```python
from build123d import *

# Parameters (mm, degrees)
SKETCH1_R                      = 1.35
BASE_FLANGE1_DEPTH             = 0.8
EDGE_FLANGE1_STRIP_W           = 7.2
EDGE_FLANGE1_STRIP_H           = 0.8
EDGE_FLANGE1_STRIP_CUT_DEPTH   = 50
EDGE_FLANGE1_STRIP_2_W         = 7.2
EDGE_FLANGE1_STRIP_2_H         = 0.8
EDGE_FLANGE1_STRIP_CUT_2_DEPTH = 55.5
EDGE_FLANGE1_DEPTH             = 50
EDGE_FLANGE1_BEND_DEPTH        = 55.5
EDGE_FLANGE4_DEPTH             = 11.5
EDGE_FLANGE4_BEND_DEPTH        = 11.5
EDGE_FLANGE5_DEPTH             = 50
EDGE_FLANGE5_BEND_DEPTH        = 55.5


# Sheet-metal steps are written as plain solids
with BuildPart() as part:
    # Sketch1 → Base-Flange1 (new body)
    with BuildSketch(Plane.XY):
        Polygon((16.25, 0), (16.25, -17), (-14.25, -17), (-14.25, -5.5), (-23.25, -5.5), (-23.25, 50), (-14.25, 50), (-14.25, 65), (16.25, 65), (16.25, 50), (21.25, 50), (21.25, 0), align=None)
        with Locations((9.737756115, -14)):
            Circle(SKETCH1_R, mode=Mode.SUBTRACT)
        with Locations((-4.262243885, -14)):
            Circle(SKETCH1_R, mode=Mode.SUBTRACT)
        with Locations((9.737756115, 62)):
            Circle(SKETCH1_R, mode=Mode.SUBTRACT)
        with Locations((-4.262243885, 62)):
            Circle(SKETCH1_R, mode=Mode.SUBTRACT)
    extrude(amount=BASE_FLANGE1_DEPTH)

    # Edge-Flange1 strip (across the edge) → Edge-Flange1 strip cut (cut)
    with BuildSketch(Plane(origin=(21.25, 50, 0), x_dir=(-1, 0, 0), z_dir=(0, -1, 0))):
        with Locations((-1.6, -0.4)):
            Rectangle(EDGE_FLANGE1_STRIP_W, EDGE_FLANGE1_STRIP_H)
    extrude(amount=EDGE_FLANGE1_STRIP_CUT_DEPTH, mode=Mode.SUBTRACT)

    # Edge-Flange1 strip 2 (across the edge) → Edge-Flange1 strip cut 2 (cut)
    with BuildSketch(Plane(origin=(-23.25, -5.5, 0), x_dir=(1, 0, 0), z_dir=(0, 1, 0))):
        with Locations((-1.6, -0.4)):
            Rectangle(EDGE_FLANGE1_STRIP_2_W, EDGE_FLANGE1_STRIP_2_H)
    extrude(amount=EDGE_FLANGE1_STRIP_CUT_2_DEPTH, mode=Mode.SUBTRACT)

    # Edge-Flange1 section (across the edge) → Edge-Flange1 (add)
    with BuildSketch(Plane(origin=(21.25, 50, 0), x_dir=(-1, 0, 0), z_dir=(0, -1, 0))):
        with BuildLine():
            Line((-0.8, 2), (-0.8, 13.5))
            Line((-0.8, 13.5), (0, 13.5))
            Line((0, 13.5), (0, 2))
            ThreePointArc((0, 2), (0.585786438, 0.585786438), (2, 0))
            Line((2, 0), (2, -0.8))
            ThreePointArc((2, -0.8), (0.020101013, 0.020101013), (-0.8, 2))
        make_face()
    extrude(amount=EDGE_FLANGE1_DEPTH)

    # Edge-Flange1 section 2 (across the edge) → Edge-Flange1 bend (add)
    with BuildSketch(Plane(origin=(-23.25, -5.5, 0), x_dir=(1, 0, 0), z_dir=(0, 1, 0))):
        with BuildLine():
            Line((-0.8, 2), (-0.8, 13.5))
            Line((-0.8, 13.5), (0, 13.5))
            Line((0, 13.5), (0, 2))
            ThreePointArc((0, 2), (0.585786438, 0.585786438), (2, 0))
            Line((2, 0), (2, -0.8))
            ThreePointArc((2, -0.8), (0.020101013, 0.020101013), (-0.8, 2))
        make_face()
    extrude(amount=EDGE_FLANGE1_BEND_DEPTH)

    # Edge-Flange4 section (across the edge) → Edge-Flange4 (add)
    with BuildSketch(Plane(origin=(21.25, 52, -2), x_dir=(0, -1, 0), z_dir=(0, 0, -1))):
        with BuildLine():
            Line((-0.8, 2), (-0.8, 20))
            Line((-0.8, 20), (0, 20))
            Line((0, 20), (0, 2))
            ThreePointArc((0, 2), (0.585786438, 0.585786438), (2, 0))
            Line((2, 0), (2, -0.8))
            ThreePointArc((2, -0.8), (0.020101013, 0.020101013), (-0.8, 2))
        make_face()
    extrude(amount=EDGE_FLANGE4_DEPTH)

    # Edge-Flange4 section 2 (across the edge) → Edge-Flange4 bend (add)
    with BuildSketch(Plane(origin=(-23.25, 52, -13.5), x_dir=(0, -1, 0), z_dir=(0, 0, 1))):
        with BuildLine():
            Line((-0.8, 2), (-0.8, 20))
            Line((-0.8, 20), (0, 20))
            Line((0, 20), (0, 2))
            ThreePointArc((0, 2), (0.585786438, 0.585786438), (2, 0))
            Line((2, 0), (2, -0.8))
            ThreePointArc((2, -0.8), (0.020101013, 0.020101013), (-0.8, 2))
        make_face()
    extrude(amount=EDGE_FLANGE4_BEND_DEPTH)

    # Edge-Flange5 section (across the edge) → Edge-Flange5 (add)
    with BuildSketch(Plane(origin=(21.25, 50, -15.5), x_dir=(0, 0, 1), z_dir=(0, -1, 0))):
        with BuildLine():
            Line((-0.8, 2), (-0.8, 10))
            Line((-0.8, 10), (0, 10))
            Line((0, 10), (0, 2))
            ThreePointArc((0, 2), (0.585786438, 0.585786438), (2, 0))
            Line((2, 0), (2, -0.8))
            ThreePointArc((2, -0.8), (0.020101013, 0.020101013), (-0.8, 2))
        make_face()
    extrude(amount=EDGE_FLANGE5_DEPTH)

    # Edge-Flange5 section 2 (across the edge) → Edge-Flange5 bend (add)
    with BuildSketch(Plane(origin=(-23.25, -5.5, -15.5), x_dir=(0, 0, 1), z_dir=(0, 1, 0))):
        with BuildLine():
            Line((-0.8, 2), (-0.8, 10))
            Line((-0.8, 10), (0, 10))
            Line((0, 10), (0, 2))
            ThreePointArc((0, 2), (0.585786438, 0.585786438), (2, 0))
            Line((2, 0), (2, -0.8))
            ThreePointArc((2, -0.8), (0.020101013, 0.020101013), (-0.8, 2))
        make_face()
    extrude(amount=EDGE_FLANGE5_BEND_DEPTH)


solid = part.part
```
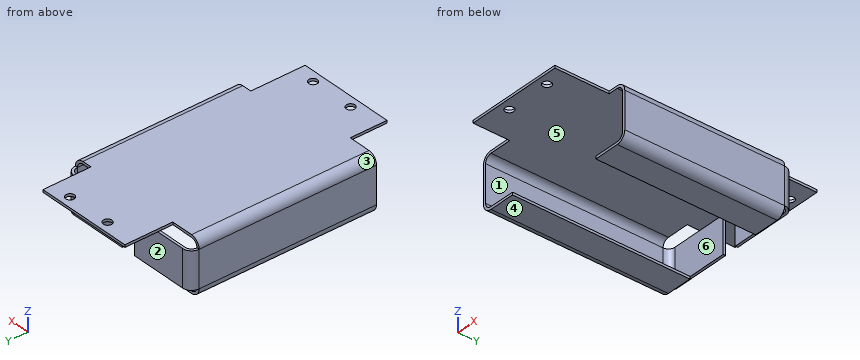
Work out the finished part from the listing and answer in its coordinate system (mm). Face numbers are marked on the shaded views. A direction names the side the tool comes from. Give positions to 0.01 mm unless a question says otherwise; leave off trailing zeros. Loops run counter-clockwise (first coordinate to the right, second up) from the corner with the lowest first, then second, coordinate; pieces in that order, holes last. Notation, with made-up numbers: (61, 30) -> (114, 30) arc R10 cw to (114, 35) -> close; hole circle Ø6 at (-4.5, 84.25). An arc over 180 degrees is marked (long way). Use CSV: the item, a comma, the result in double quotes.
1. A tool of negligible diameter and unlimited length cuts with its end or side. For the marked faces 4, 5 and 6, from which of +Z, -Z, +X, -X, +Y, -Y can it reach the whole face along a straight path? Write none if from no direction.
Found:
face 4,"-Z, +X, -X, +Y, -Y"
face 5,"+Y, -Y"
face 6,"-Z, -Y"
2. The part is cut by section A-A (x = -10.5). Write down the section's boundary in (y, z), then the cut area to 3 significant figures.
Found:
outline,"(-17, 0) -> (65, 0) -> (65, 0.8) -> (-17, 0.8) -> close; (52, -13.5) -> (52.8, -13.5) -> (52.8, -2) -> (52, -2) -> close"
area,"74.8 mm^2"
3. Straight lines are drawn through the part: line 1 (X direction, y = 47.5, z = -4.5); line 2 (Y direction, x = 6.5, z = -6.25); line 3 (Z direction, x = 7, y = 49). For each, find the intervals that lie inside material, in ascending order.
Found:
line 1,"-24.05 to -23.25, 21.25 to 22.05"
line 2,"52 to 52.8"
line 3,"0 to 0.8"
4. The mould has two halves that part along Z. Classify the marked faces 1, 2 and 3: +Z half, -Z half, draft (parallel to the pull), parting line (faces both ways), or undercut.
Found:
face 1,"undercut"
face 2,"draft"
face 3,"+Z half"
5. The part is cut by section B-B (y = 62). Write down the section's boundary in (x, z), then the cut area to 3 significant figures.
Found:
outline,"(-14.25, 0) -> (-5.61, 0) -> (-5.61, 0.8) -> (-14.25, 0.8) -> close; (-2.91, 0) -> (8.39, 0) -> (8.39, 0.8) -> (-2.91, 0.8) -> close; (11.09, 0) -> (16.25, 0) -> (16.25, 0.8) -> (11.09, 0.8) -> close"
area,"20.1 mm^2"
6. The part is cut by section C-C (x = -18). Write down the section's boundary in (y, z), then the cut area to 3 significant figures.
Found:
outline,"(-5.5, -16.3) -> (50, -16.3) -> (50, -15.5) -> (-5.5, -15.5) -> close; (-5.5, 0) -> (50, 0) -> (50, 0.8) -> (-5.5, 0.8) -> close; (52, -13.5) -> (52.8, -13.5) -> (52.8, -2) -> (52, -2) -> close"
area,"98.0 mm^2"
7. The part is cut by section D-D (z = -11.75). Write down the section's boundary in (x, y).
Found:
outline,"(-24.05, -5.5) -> (-23.25, -5.5) -> (-23.25, 50) arc R2 cw to (-21.25, 52) -> (-3.25, 52) -> (-3.25, 52.8) -> (-21.25, 52.8) arc R2.8 ccw to (-24.05, 50) -> close; (1.25, 52) -> (19.25, 52) arc R2 cw to (21.25, 50) -> (21.25, 0) -> (22.05, 0) -> (22.05, 50) arc R2.8 ccw to (19.25, 52.8) -> (1.25, 52.8) -> close"
8. Flat-ended cylindrical pins translate along their axes: pin 1 Ø2 at (x, z) = (17, -15) entering from +Y; pin 2 Ø12 at (x, y) = (-6.5, 28.5) entering from -Z; pin 3 Ø6 at (x, z) = (13.5, -9.5) entering from +Y; pin 4 Ø10 at (x, y) = (7, 13.5) entering from -Z. Find the tip coordinate at first contact, or state that the pin passes through.
Found:
pin 1,"y = 50"
pin 2,"z = 0"
pin 3,"y = 52.8"
pin 4,"z = -16.3"
